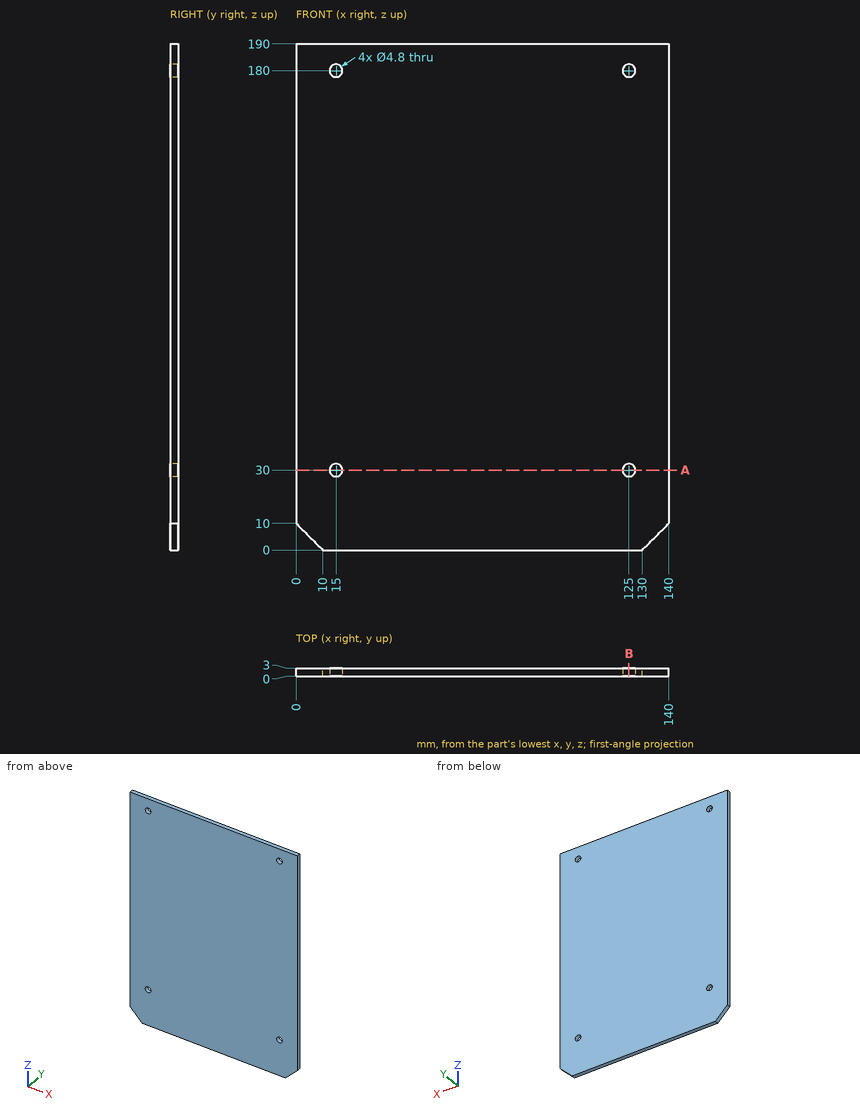
Answer from the drawing. Dimensions are ordinates in mm from the lowest x, y and z of the part. Round coordinates to 2 decimals unless told otherwise and drop trailing zeros. Write each loop counter-clockwise with the first axis right and the second up, starting at its lowest first coordinate (ties: lowest second). Pieces come first, ordered by that corner, then holes.
1. Straight lines are drawn through the part: L1, parallel to X at y = 0.85, z = 30; L2, parallel to Z at x = 15, y = 1.8; L3, parallel to X at y = 0.35, z = 179.5. For each, find the intervals that lie inside material, in ascending order.
2. The part is cut by section B-B, the plane x = 125. Determine the outline of the cut face in (y, z).
3. Given pin 1 Ø1.5 at (x, y) = (44.5, 1) entering from -Z, flat-ended and moving along its own axis, determine where the tip first touches the part or whether it passes through.
4. The part is cut by section A-A, the plane z = 30. Determine the outline of the cut face in (x, y).
Values:
1. L1: x = 0 to 12.6, 17.4 to 122.6, 127.4 to 140
1. L2: z = 0 to 27.6, 32.4 to 177.6, 182.4 to 190
1. L3: x = 0 to 12.65, 17.35 to 122.65, 127.35 to 140
2. outline: (0, 0) - (3, 0) - (3, 27.6) - (0, 27.6) - close; (0, 32.4) - (3, 32.4) - (3, 177.6) - (0, 177.6) - close; (0, 182.4) - (3, 182.4) - (3, 190) - (0, 190) - close
3. pin 1: stops at z = 0
4. outline: (0, 0) - (12.6, 0) - (12.6, 3) - (0, 3) - close; (17.4, 0) - (122.6, 0) - (122.6, 3) - (17.4, 3) - close; (127.4, 0) - (140, 0) - (140, 3) - (127.4, 3) - close
